Autodesk Inventor part; units mm, degrees
ref_plane "YZ Plane" through (0, 0, 0) normal (1, 0, 0) x (0, 1, 0)
ref_plane "XZ Plane" through (0, 0, 0) normal (0, 1, 0) x (-1, 0, 0)
ref_plane "XY Plane" through (0, 0, 0) normal (0, 0, 1) x (1, 0, 0)
sketch "Sketch1" plane through (0, 0, 0) normal (0, 1, 0) x (-1, 0, 0)
  line L0 (190, 210) -> (190, -210)
  line L1 (190, -210) -> (-150, -210)
  line L2 (-150, -210) -> (-150, 210)
  line L3 (-150, -190) -> (170, -190)
  line L4 (170, -190) -> (170, 190)
  line L5 (-150, -200) -> (180, -200)
  line L6 (180, -200) -> (180, 200)
  line L7 (190, -210) -> (190, -90)
  line L8 (190, -90) -> (-150, -90)
  line L9 (170, 190) -> (170, 210)
  line L10 (180, 200) -> (180, 210)
  line L11 (170, 210) -> (190, 210)
  line L12 (190, -90) -> (190, -100)
  line L13 (190, -100) -> (-150, -100)
  line L14 (190, -100) -> (190, -110)
  line L15 (190, -110) -> (-150, -110)
  circle A0 centre (180, 200) radius 2.5
  circle A1 centre (180, -100) radius 2.5
  circle A2 centre (20, -100) radius 2.5
  circle A3 centre (180, 100) radius 2.5
  circle A4 centre (180, 0) radius 2.5
  line L16 (0, 0) -> (0, 25.5231)
  circle A5 centre (160, -200) radius 2.5
  line L17 (-150, -200) -> (-140, -200)
  line L18 (-140, -200) -> (-130, -200)
  line L19 (-130, -200) -> (-130, 210)
  line L20 (-130, 210) -> (-150, 210)
  circle A6 centre (-140, -100) radius 2.5
  circle A7 centre (-140, 0) radius 2.5
  circle A8 centre (-140, 100) radius 2.5
  circle A9 centre (-140, 200) radius 2.5
  circle A10 centre (20, -200) radius 2.5
  line L21 (20, -200) -> (-120, -200)
  circle A11 centre (-120, -200) radius 2.5
  point P0 (170, -90)
  point P1 (180, -90)
  point P2 (-130, -90)
  point P3 (-130, -190)
  point P4 (180, 2.5)
  point P5 (180, -2.5)
  point P6 (180, 202.5)
  point P7 (180, 197.5)
  point P8 (180, 102.5)
  point P9 (180, 97.5)
  dimension "d0" = 340
  dimension "d1" = 420
  dimension "d2" = 20
  dimension "d3" = 10
  dimension "d4" = 120
  dimension "d5" = 10
  dimension "d6" = 10
  dimension "d7" = 5
  dimension "d9" = 5
  dimension "d11" = 5
  dimension "d12" = 5
  dimension "d13" = 5
  dimension "d15" = 5
  dimension "d25" = 10
  dimension "d26" = 10
  dimension "d27" = 5
  dimension "d30" = 5
  dimension "d31" = 140
  dimension "d32" = 5
extrude "Extrusion1" add sketch "Sketch1" along normal blind 3 contours L0 L8 L6 A4 A3 A0 L10 L11 | L0 L13 A1 L6 L8 | L10 A0 L6 A3 A4 L8 L4 L9 L11 | L0 L15 L6 A1 L13 | L6 A1 L13 L4 L8 | L0 L1 L2 L5 A11 A10 A5 L6 L15 | L4 L13 A2 L19 L8 | L15 L4 L13 A1 L6 | L6 L5 A5 A10 A11 L19 L3 L4 L15 | L4 L15 L19 L13 A2 | L19 L13 A6 L2 L8 | L8 L2 L20 L19 | L4 L3 L19 L15 | L19 L15 L2 L13 A6 | L2 L3 L19 L5 | L19 L3 L2 L15 | A6 L13 | L13 A6 | A10 L5 | L5 A10 | A11 L5 | L5 A11
sketch "Sketch3" plane through (0, 3, 0) normal (0, 1, 0) x (1, 0, 0)
  circle A0 centre (-180, -100) radius 2.5
  circle A1 centre (-20, 100) radius 2.5
  circle A2 centre (-160, 200) radius 2.5
  circle A3 centre (-180, 100) radius 2.5
  circle A4 centre (140, 0) radius 2.5
  circle A5 centre (140, -100) radius 2.5
  circle A6 centre (140, -200) radius 2.5
  circle A7 centre (-180, -200) radius 2.5
  line L0 (-190, 210) -> (-190, -210)
  line L1 (-190, -210) -> (-170, -210)
  line L2 (-170, -210) -> (-170, 90)
  line L3 (-170, 90) -> (130, 90)
  line L4 (130, 90) -> (130, -210)
  line L5 (130, -210) -> (150, -210)
  line L6 (150, -210) -> (150, 210)
  line L7 (150, 210) -> (-190, 210)
  circle A8 centre (-180, 0) radius 2.5
  circle A9 centre (-20, 200) radius 2.5
  circle A10 centre (120, 200) radius 2.5
  circle A11 centre (-180, -100) radius 2.5
  circle A12 centre (-20, 100) radius 2.5
  circle A13 centre (-160, 200) radius 2.5
  circle A14 centre (-180, 100) radius 2.5
  circle A15 centre (140, 0) radius 2.5
  circle A16 centre (140, -100) radius 2.5
  circle A17 centre (140, -200) radius 2.5
  circle A18 centre (-180, -200) radius 2.5
  line L8 (-190, 210) -> (-190, -210)
  line L9 (-190, -210) -> (-170, -210)
  line L10 (-170, -210) -> (-170, 90)
  line L11 (-170, 90) -> (130, 90)
  line L12 (130, 90) -> (130, -210)
  line L13 (130, -210) -> (150, -210)
  line L14 (150, -210) -> (150, 210)
  line L15 (150, 210) -> (-190, 210)
  circle A19 centre (-180, 0) radius 2.5
  circle A20 centre (140, 100) radius 2.5
  point P0 (0, 0)
extrude "Extrusion3" cut sketch "Sketch3" against normal blind 3 contours A10 | A20
properties part number "CaraFrontal"
The model under review builds one solid part; all positions refer to its coordinate system, in mm. Round coordinates to 2 decimals unless told otherwise and drop trailing zeros. Order: outer loops, then holes, each group sorted by start corner. A loop starts at its lowest first (then second) coordinate and runs counter-clockwise, first axis right, second up. Notation, with made-up numbers: (47.25, 63.25) -> (105.25, 63.25) arc R15 ccw to (105.25, 86.25) -> close; hole circle Ø3 at (-30.5, 9). An arc over 180 degrees is marked (long way). Use a Markdown table: item, result.
Q1. We need section A-A on y = 2.55. State how many separate pieces and enclosed holes the cut face has, then the cut area to 3 significant figures.
Values:
| item | result |
|---|---|
| separate pieces | 1 |
| enclosed holes | 11 |
| area | 52,600 mm^2 |
Q2. Clearance check with flat-ended pins moving along their axes: P1, Ø4, axis at x = -20, z = -100, coming from the +Y side; P2, Ø1.5, axis at x = 95, y = 1.5, coming from the +Z side. State where each tip first meets the part, or that it passes through.
Values:
| item | result |
|---|---|
| P1 | passes through |
| P2 | stops at z = -90 |
Q3. We need section B-B on z = 160.5. Write out the cut boundary in (x, y), then the cut area to 3 significant figures.
Values:
| item | result |
|---|---|
| outline | (-190, 0) -> (-170, 0) -> (-170, 3) -> (-190, 3) -> close; (130, 0) -> (150, 0) -> (150, 3) -> (130, 3) -> close |
| area | 120 mm^2 |
Q4. We need section C-C on x = -83.5. Write out the cut boundary in (y, z), then the cut area to 3 significant figures.
Values:
| item | result |
|---|---|
| outline | (0, -210) -> (3, -210) -> (3, -90) -> (0, -90) -> close |
| area | 360 mm^2 |
Q5. For line 1 (X direction, y = 2.45, z = -100); line 2 (Z direction, x = 140, y = 1.3); line 3 (X direction, y = 0.65, z = 173), list the stretches that pass through material, from the lowest coordinate up.
Values:
| item | result |
|---|---|
| line 1 | x = -190 to -182.5, -177.5 to -22.5, -17.5 to 137.5, 142.5 to 150 |
| line 2 | z = -210 to -102.5, -97.5 to -2.5, 2.5 to 97.5, 102.5 to 197.5, 202.5 to 210 |
| line 3 | x = -190 to -170, 130 to 150 |
